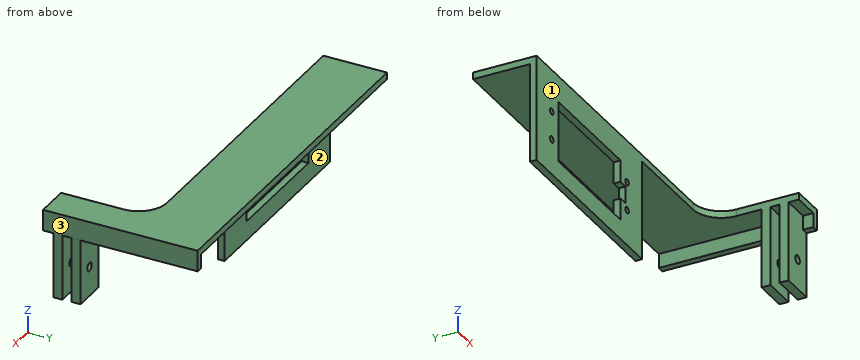
from build123d import *

# Parameters (mm, degrees)
SKETCH1_W               = 70
SKETCH1_H               = 35
BOSS_EXTRUDE1_DEPTH     = 2.4
SKETCH2_R               = 1.13
SKETCH2_W               = 40
SKETCH2_H               = 20
CUT_EXTRUDE1_DEPTH      = 2.4
SKETCH4_W               = 4
SKETCH4_H               = 6
CUT_EXTRUDE2_DEPTH      = 2.4
CUT_EXTRUDE3_DEPTH      = 134.373649476
CUT_EXTRUDE3_DEPTH_BACK = 134.373649476
SKETCH7_W               = 41.3
SKETCH7_H               = 21.3
SKETCH7_W_2             = 40
SKETCH7_H_2             = 20
BOSS_EXTRUDE2_DEPTH     = 2.4
SKETCH9_W               = 11.879910587
SKETCH9_H               = 3.175
SKETCH9_W_2             = 12
BOSS_EXTRUDE3_DEPTH     = 28
SKETCH10_R              = 1.4732
CUT_EXTRUDE4_DEPTH      = 30
FILLET1_R               = 10
SKETCH11_W              = 5
SKETCH11_H              = 54.4
BOSS_EXTRUDE4_DEPTH     = 2.4


with BuildPart() as part:
    # Sketch1 → Boss-Extrude1 (new body)
    with BuildSketch(Plane(origin=(0, 0, 0), x_dir=(1, 0, 0), z_dir=(0, 1, 0))):
        with Locations((92.522946176, 21.495750708)):
            Rectangle(SKETCH1_W, SKETCH1_H)
    extrude(amount=BOSS_EXTRUDE1_DEPTH)

    # Sketch2 → Cut-Extrude1 (cut)
    with BuildSketch(Plane(origin=(0, 2.4, 0), x_dir=(1, 0, 0), z_dir=(0, 1, 0))):
        with Locations(Location((67.522946176, 26.495750708, 0), (0, 0, 270))):
            Circle(SKETCH2_R)
        with Locations(Location((117.522946176, 26.495750708, 0), (0, 0, 270))):
            Circle(SKETCH2_R)
        with Locations(Location((117.522946176, 16.495750708, 0), (0, 0, 90))):
            Circle(SKETCH2_R)
        with Locations(Location((67.522946176, 16.495750708, 0), (0, 0, 90))):
            Circle(SKETCH2_R)
        with Locations((92.522946176, 21.495750708)):
            Rectangle(SKETCH2_W, SKETCH2_H)
    extrude(amount=-CUT_EXTRUDE1_DEPTH, mode=Mode.SUBTRACT)

    # Sketch4 → Cut-Extrude2 (cut)
    with BuildSketch(Plane(origin=(0, 2.4, 0), x_dir=(1, 0, 0), z_dir=(0, 1, 0))):
        with Locations((114.522946176, 21.495750708)):
            Rectangle(SKETCH4_W, SKETCH4_H)
    extrude(amount=-CUT_EXTRUDE2_DEPTH, mode=Mode.SUBTRACT)

    # Sketch7 → Cut-Extrude3 (cut, two sides: drawn at the far end of the back side and taken through both)
    with BuildSketch(Plane(origin=(0, 2.4, 0), x_dir=(1, 0, 0), z_dir=(0, 1, 0)).offset(-CUT_EXTRUDE3_DEPTH_BACK)):
        with Locations((92.522946176, 21.495750708)):
            Rectangle(SKETCH7_W, SKETCH7_H)
        with Locations((92.522946176, 21.495750708)):
            Rectangle(SKETCH7_W_2, SKETCH7_H_2, mode=Mode.SUBTRACT)
    extrude(amount=CUT_EXTRUDE3_DEPTH + CUT_EXTRUDE3_DEPTH_BACK, mode=Mode.SUBTRACT)

    # Sketch8 → Boss-Extrude2 (add)
    with BuildSketch(Plane.XY.offset(-3.995750708)):
        Polygon((57.522946176, 22.4), (183.172946176, 22.4), (183.172946176, -32), (171.172946176, -32), (171.172946176, 0), (57.522946176, 0), align=None)
    extrude(amount=BOSS_EXTRUDE2_DEPTH)

    # Sketch9 → Boss-Extrude3 (add)
    with BuildSketch(Plane(origin=(0, 0, -3.995750708), x_dir=(-1, 0, 0), z_dir=(0, 0, -1))):
        with Locations((-177.11290147, -20.4125)):
            Rectangle(SKETCH9_W, SKETCH9_H)
        with Locations((-177.172946176, -26.7625)):
            Rectangle(SKETCH9_W_2, SKETCH9_H)
    extrude(amount=BOSS_EXTRUDE3_DEPTH)

    # Sketch10 → Cut-Extrude4 (cut)
    with BuildSketch(Plane.XZ.offset(28.35)):
        with Locations(Location((177.172946176, -21.495750708, 0), (0, 0, 270))):
            Circle(SKETCH10_R)
    extrude(amount=-CUT_EXTRUDE4_DEPTH, mode=Mode.SUBTRACT)

    # Fillet1
    fillet1_edges = [part.edges().sort_by_distance(p)[0] for p in [
        (171.172946176, 0, -2.795750708),
    ]]
    fillet(fillet1_edges, radius=FILLET1_R)

    # Sketch11 → Boss-Extrude4 (add)
    with BuildSketch(Plane(origin=(183.172946176, 0, 0), x_dir=(0, 0, -1), z_dir=(1, 0, 0))):
        with Locations((6.495750708, -4.8)):
            Rectangle(SKETCH11_W, SKETCH11_H)
    extrude(amount=-BOSS_EXTRUDE4_DEPTH)


solid = part.part
Geometry check sheet. Reference: the model listing, model coordinates, mm. Face numbers are marked on the shaded views. A direction names the side the tool comes from. Round coordinates to 2 decimals unless told otherwise and drop trailing zeros. Order: outer loops, then holes, each group sorted by start corner. A loop starts at its lowest first (then second) coordinate and runs counter-clockwise, first axis right, second up. Notation, with made-up numbers: M 61,53.25 L 76,53.25 A5 cw 76,57.25 Z; hole C 28.5,13.25 d10. An arc over 180 degrees is marked long. Write each question's results on one line, items separated by ' | '. Start each with the question number.
1. Material ranges on L1, parallel to Z at x = 64.5, y = 7; L2, parallel to Y at x = 119.5, z = -24; L3, parallel to Y at x = 102, z = -3, recorded low to high. Write a range as from..to.
2. Cross-section at D-D on x = 173. Record the boundary of the cut face in (y, z) (3 decimals).
3. Cross-section at B-B on z = -6.5. Record the boundary of the cut face in (x, y) (3 decimals).
4. Cross-section at A-A on x = 98. Record the boundary of the cut face in (y, z).
5. Set-up check for the marked faces 1, 2 and 3: record each of +Z, -Z, +X, -X, +Y, -Y from which the full face is reachable in a straight line by a thin tool's end or side.
6. Cross-section at C-C on y = -20.5. Record the boundary of the cut face in (x, z).
7. Go/stop test with flat-tipped pins: P1, Ø1.6, axis at x = 177, y = -20.5, coming from the -Z side; P2, Ø13, axis at x = 176.5, z = -19, coming from the +Y side (3 decimals); P3, Ø13, axis at x = 178, z = -20.5, coming from the -Y side. Record where each tip stops, or that it passes through.
Resolved:
1) L1: -4..-1.6 | L2: 0..2.4 | L3: 0..22.4
2) outline: M -32,-3.996 L -28.35,-3.996 L -28.35,-31.996 L -25.175,-31.996 L -25.175,-3.996 L -22,-3.996 L -22,-31.996 L -18.825,-31.996 L -18.825,-3.996 L 22.4,-3.996 L 22.4,-1.596 L -32,-1.596 Z
3) outline: M 57.523,0 L 127.523,0 L 127.523,2.4 L 57.523,2.4 Z; M 171.173,-28.35 L 180.773,-28.35 L 180.773,-32 L 183.173,-32 L 183.173,22.4 L 180.773,22.4 L 180.773,-18.825 L 171.173,-18.825 L 171.173,-22 L 180.773,-22 L 180.773,-25.175 L 171.173,-25.175 Z
4) outline: M 0,-39 L 2.4,-39 L 2.4,-32.15 L 0,-32.15 Z; M 0,-10.85 L 2.4,-10.85 L 2.4,-4 L 22.4,-4 L 22.4,-1.6 L 0,-1.6 Z
5) face 1: +Z, -Z, -X, -Y | face 2: -Z, -X, +Y | face 3: +Z, -Z, +X, +Y, -Y
6) outline: M 171.17,-32 L 183.05,-32 L 183.05,-9 L 183.17,-9 L 183.17,-1.6 L 171.17,-1.6 Z; hole C 177.17,-21.5 d2.95
7) P1: z = -32 | P2: y = -18.825 | P3: y = -28.35
